The listing builds one solid part. Answer for the finished solid, in the listing's coordinates (mm). Give positions to 0.01 mm unless a question says otherwise; leave off trailing zeros. Write each loop counter-clockwise with the first axis right and the second up, starting at its lowest first coordinate (ties: lowest second). Pieces come first, ordered by that corner, then holes. Notation, with made-up numbers: M -32,77 L 16,77 A22 cw 16,110 Z; hole C 46.25,21.5 d3. An arc over 180 degrees is marked long. Return JSON: item names as keys, results as strings.
from build123d import *

# Parameters (mm, degrees)
SKIZZE1_W                        = 100
SKIZZE1_H                        = 2.5
VERRUNDUNG1_R                    = 0.75
VERRUNDUNG2_R                    = 0.75
F_3_5_3_5_DURCHMESSER_BOHRUNG1_D = 3.5


with BuildPart() as part:
    # Skizze1 → Rotation1 (revolve)
    with BuildSketch(Plane.XY):
        with Locations((-50, 1.25)):
            Rectangle(SKIZZE1_W, SKIZZE1_H)
    revolve(axis=Axis((0, 0, 0), (-1, 0, 0)))

    # Verrundung1
    verrundung1_edges = [part.edges().sort_by_distance(p)[0] for p in [
        (-100, -2.5, 0),
    ]]
    fillet(verrundung1_edges, radius=VERRUNDUNG1_R)

    # Verrundung2
    verrundung2_edges = [part.edges().sort_by_distance(p)[0] for p in [
        (0, -2.5, 0),
    ]]
    fillet(verrundung2_edges, radius=VERRUNDUNG2_R)

    # Ø3.5 (3.5) Durchmesser Bohrung1 (through all)
    with Locations(Plane(origin=(-4, 0.063040866, 2.499205043), x_dir=(0, 0.999682017384, -0.025216346285), z_dir=(0, 0.025216346285, 0.999682017384))):
        with Locations((0, 0)):
            Hole(F_3_5_3_5_DURCHMESSER_BOHRUNG1_D / 2)


solid = part.part
Item 1: Given pin 1 Ø3 at (x, z) = (-53, 1.5) entering from -Y; pin 2 Ø2 at (x, z) = (-28, -2) entering from +Y, each flat-ended and moving along its own axis, determine where each tip first touches the part or whether it passes through.
Geometry results:
{"pin 1": "stops at y = -2.5", "pin 2": "stops at y = 2.29"}
Item 2: Determine the mould class of faces 1 (the flat face through (-100, 0, 0)), 2 (the cylindrical face through (-3.33, -1.617, 0.006)), 3 (the cylindrical face through (-49.31, 2.385, -0.751)) for opening direction Y: +Y half, -Y half, draft (parallel to the pull), parting line (faces both ways), or undercut.
Geometry results:
{"face 1": "draft", "face 2": "undercut", "face 3": "parting line"}
Item 3: A cutting plane is placed at A-A, the plane x = -55.5. Write down the section's boundary in (y, z).
Geometry results:
{"outline": "C 0,0 d5"}
Item 4: Find the intervals of material crossed by line 1 (X direction, y = 0.25, z = -0.4); line 2 (X direction, y = -1.3, z = -1.7); line 3 (Z direction, x = -6, y = -0.2), in increasing order.
Geometry results:
{"line 1": "x = -100 to -5.73, -2.27 to 0", "line 2": "x = -99.89 to -5.22, -2.78 to -0.11", "line 3": "z = -2.49 to 2.49"}
